```python
from build123d import *

# Parameters (mm, degrees)
BOSS_EXTRUDE1_DEPTH  = 150
CUT_EXTRUDE1_DEPTH   = 152.20350525
LPATTERN1_COUNT      = 6
LPATTERN1_PITCH      = 25
MIRROR2_COPY_1_DEPTH = 152.20350525
MIRROR2_COPY_2_DEPTH = 152.20350525
MIRROR2_COPY_3_DEPTH = 152.20350525
MIRROR2_COPY_4_DEPTH = 152.20350525
MIRROR2_COPY_5_DEPTH = 152.20350525


with BuildPart() as part:
    # Sketch1 → Boss-Extrude1 (new body)
    with BuildSketch(Plane.XY):
        Polygon((0, 0), (13.5, 0), (13.5, 6.5), (17.5, 6.5), (17.5, 7.5), (12.5, 7.5), (12.5, 1), (0, 1), align=None)
    boss_extrude1 = extrude(amount=BOSS_EXTRUDE1_DEPTH)

    # Sketch2 → Cut-Extrude1 (cut, through all)
    with BuildSketch(Plane(origin=(0, 0, 0), x_dir=(1, 0, 0), z_dir=(0, 1, 0))):
        with BuildLine():
            Line((3.1, -8.1), (3.1, -16.9))
            ThreePointArc((3.1, -16.9), (0, -20), (-3.1, -16.9))
            Line((-3.1, -16.9), (-3.1, -8.1))
            ThreePointArc((-3.1, -8.1), (0, -5), (3.1, -8.1))
        make_face()
    cut_extrude1 = extrude(amount=CUT_EXTRUDE1_DEPTH, mode=Mode.SUBTRACT)

    # LPattern1: Cut-Extrude1 ×6
    with Locations(*[(0, 0, i * LPATTERN1_PITCH) for i in range(1, LPATTERN1_COUNT)]):
        add(cut_extrude1, mode=Mode.SUBTRACT)

    # Mirror2: Boss-Extrude1, Cut-Extrude1 across plane
    add(boss_extrude1.mirror(Plane(origin=(0, 0, 0), x_dir=(0, 0, 1), z_dir=(1, 0, 0))))
    add(cut_extrude1.mirror(Plane(origin=(0, 0, 0), x_dir=(0, 0, 1), z_dir=(1, 0, 0))), mode=Mode.SUBTRACT)

    # Mirror2 copy 1 sketch → Mirror2 copy 1 (cut, through all)
    with BuildSketch(Plane(origin=(0, 0, 25), x_dir=(-1, 0, 0), z_dir=(0, 1, 0))):
        with BuildLine():
            Line((3.1, 8.1), (3.1, 16.9))
            ThreePointArc((3.1, 16.9), (0, 20), (-3.1, 16.9))
            Line((-3.1, 16.9), (-3.1, 8.1))
            ThreePointArc((-3.1, 8.1), (0, 5), (3.1, 8.1))
        make_face()
    extrude(amount=MIRROR2_COPY_1_DEPTH, mode=Mode.SUBTRACT)

    # Mirror2 copy 2 sketch → Mirror2 copy 2 (cut, through all)
    with BuildSketch(Plane(origin=(0, 0, 50), x_dir=(-1, 0, 0), z_dir=(0, 1, 0))):
        with BuildLine():
            Line((3.1, 8.1), (3.1, 16.9))
            ThreePointArc((3.1, 16.9), (0, 20), (-3.1, 16.9))
            Line((-3.1, 16.9), (-3.1, 8.1))
            ThreePointArc((-3.1, 8.1), (0, 5), (3.1, 8.1))
        make_face()
    extrude(amount=MIRROR2_COPY_2_DEPTH, mode=Mode.SUBTRACT)

    # Mirror2 copy 3 sketch → Mirror2 copy 3 (cut, through all)
    with BuildSketch(Plane(origin=(0, 0, 75), x_dir=(-1, 0, 0), z_dir=(0, 1, 0))):
        with BuildLine():
            Line((3.1, 8.1), (3.1, 16.9))
            ThreePointArc((3.1, 16.9), (0, 20), (-3.1, 16.9))
            Line((-3.1, 16.9), (-3.1, 8.1))
            ThreePointArc((-3.1, 8.1), (0, 5), (3.1, 8.1))
        make_face()
    extrude(amount=MIRROR2_COPY_3_DEPTH, mode=Mode.SUBTRACT)

    # Mirror2 copy 4 sketch → Mirror2 copy 4 (cut, through all)
    with BuildSketch(Plane(origin=(0, 0, 100), x_dir=(-1, 0, 0), z_dir=(0, 1, 0))):
        with BuildLine():
            Line((3.1, 8.1), (3.1, 16.9))
            ThreePointArc((3.1, 16.9), (0, 20), (-3.1, 16.9))
            Line((-3.1, 16.9), (-3.1, 8.1))
            ThreePointArc((-3.1, 8.1), (0, 5), (3.1, 8.1))
        make_face()
    extrude(amount=MIRROR2_COPY_4_DEPTH, mode=Mode.SUBTRACT)

    # Mirror2 copy 5 sketch → Mirror2 copy 5 (cut, through all)
    with BuildSketch(Plane(origin=(0, 0, 125), x_dir=(-1, 0, 0), z_dir=(0, 1, 0))):
        with BuildLine():
            Line((3.1, 8.1), (3.1, 16.9))
            ThreePointArc((3.1, 16.9), (0, 20), (-3.1, 16.9))
            Line((-3.1, 16.9), (-3.1, 8.1))
            ThreePointArc((-3.1, 8.1), (0, 5), (3.1, 8.1))
        make_face()
    extrude(amount=MIRROR2_COPY_5_DEPTH, mode=Mode.SUBTRACT)


solid = part.part
```
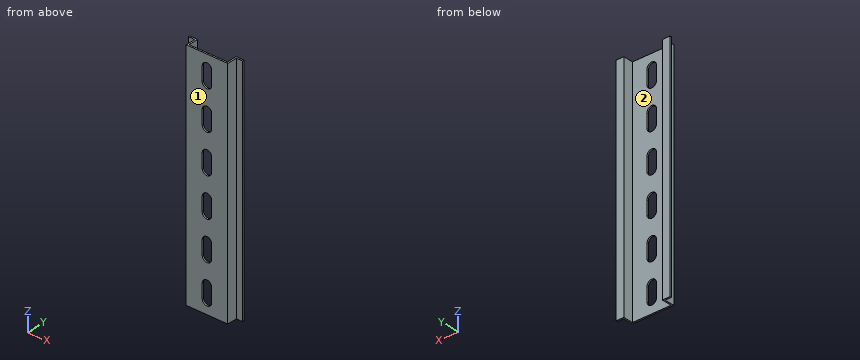
Can you work these out from the model? Positions are in its coordinate system, mm. Face numbers are marked on the shaded views. Give positions to 0.01 mm unless a question says otherwise; leave off trailing zeros. Order: outer loops, then holes, each group sorted by start corner. A loop starts at its lowest first (then second) coordinate and runs counter-clockwise, first axis right, second up. Notation, with made-up numbers: M 36.5,-39.75 L 69.5,-39.75 A16 ccw 69.5,-31.75 Z; hole C 18,-27.5 d5. An arc over 180 degrees is marked long. Write item = value, one per line. Start each with the question number.
Q1. I need wall thicknesses on probe 1 along X at (y, z) = (4.25, 20); probe 2 along X at (y, z) = (7, 27); probe 3 along Y at (x, z) = (-11.5, 79). Which ranges of each line are inside material? Lowest first, please. Write a range as [from, to].
Q2. Suppose I cut it at D-D (x = -9). Write out the boundary of the cut face in (y, z).
Q3. Will these pins go through, and if not, where does the flat tip stop? pin 1 Ø12 at (x, z) = (3, 71.5) entering from +Y; pin 2 Ø0.5 at (y, z) = (0.5, 113.5) entering from +X; pin 3 Ø0.8 at (y, z) = (0.5, 63) entering from -X.
Q4. Suppose I cut it at C-C (z = 48). Write out the boundary of the cut face in (x, y), plus the area to 3 significant figures.
Q5. Suppose I cut it at A-A (y = 4.75). Write out the boundary of the cut face in (x, z).
Q6. We'd pull the mould along X, two halves only. Please class the marked faces 1 and 2: pulls with the +X half, pulls with the -X half, needs draft (parallel to the pull), parting line crosses it, or undercut.
Q7. Suppose I cut it at B-B (z = 113.5). Write out the boundary of the cut face in (x, y).
Check result:
q1.probe_1 = [-13.5, -12.5], [12.5, 13.5]
q1.probe_2 = [-17.5, -12.5], [12.5, 17.5]
q1.probe_3 = [0, 1]
q2.outline = M 0,0 L 1,0 L 1,150 L 0,150 Z
q3.pin_1 = 1
q3.pin_2 = 13.5
q3.pin_3 = -13.5
q4.outline = M -17.5,6.5 L -13.5,6.5 L -13.5,0 L 13.5,0 L 13.5,6.5 L 17.5,6.5 L 17.5,7.5 L 12.5,7.5 L 12.5,1 L -12.5,1 L -12.5,7.5 L -17.5,7.5 Z
q4.area = 48.0 mm2
q5.outline = M -13.5,0 L -12.5,0 L -12.5,150 L -13.5,150 Z; M 12.5,0 L 13.5,0 L 13.5,150 L 12.5,150 Z
q6.face_1 = needs draft
q6.face_2 = undercut
q7.outline = M -17.5,6.5 L -13.5,6.5 L -13.5,0 L -3.1,0 L -3.1,1 L -12.5,1 L -12.5,7.5 L -17.5,7.5 Z; M 3.1,0 L 13.5,0 L 13.5,6.5 L 17.5,6.5 L 17.5,7.5 L 12.5,7.5 L 12.5,1 L 3.1,1 Z
